Verification items for the finished model (mm, model axes). A direction names the side the tool comes from. Round coordinates to 2 decimals unless told otherwise and drop trailing zeros. Loops run counter-clockwise (first coordinate to the right, second up) from the corner with the lowest first, then second, coordinate; pieces in that order, holes last. Notation, with made-up numbers: (68.5, -1) -> (91.5, -1) arc R10 cw to (91.5, 6) -> close; hole circle Ø3 at (40, -5). An arc over 180 degrees is marked (long way). Write item = value, one per line.
Autodesk Inventor part; units mm, degrees
ref_plane "YZ Plane" through (0, 0, 0) normal (1, 0, 0) x (0, 1, 0)
ref_plane "XZ Plane" through (0, 0, 0) normal (0, 1, 0) x (-1, 0, 0)
ref_plane "XY Plane" through (0, 0, 0) normal (0, 0, 1) x (1, 0, 0)
sketch "Sketch1" plane through (0, 0, 0) normal (0, 1, 0) x (-1, 0, 0)
  line L0 (0, 21.535) -> (65.7, 21.535)
  line L1 (0, 21.535) -> (40.8722, -5.4921)
  line L2 (0, 21.535) -> (49, 21.535) construction
  line L3 (40.8722, -5.4921) -> (65.7, 21.535)
  line L4 (65.7, 21.535) -> (68.7, 21.535)
  line L5 (68.7, 21.535) -> (0, 21.535)
  line L6 (0, 21.535) -> (-3, 21.535)
  line L7 (40.8722, -5.4921) -> (43.3746, -7.1468)
  line L8 (65.7, 21.535) -> (38.8426, -7.7015)
  line L9 (137.4, 18.035) -> (137.4, 25.035)
  line L10 (137.4, 25.035) -> (0, 25.035)
  line L11 (0, 25.035) -> (0, 18.035)
  line L12 (0, 18.035) -> (137.4, 18.035)
  line L13 (137.4, 18.035) -> (0, 25.035) construction
  line L14 (137.4, 25.035) -> (0, 18.035) construction
  line L15 (93.1053, 46.1943) -> (87.9503, 50.9298)
  line L16 (87.9503, 50.9298) -> (38.2947, -3.1243)
  line L17 (38.2947, -3.1243) -> (43.4497, -7.8599)
  line L18 (43.4497, -7.8599) -> (93.1053, 46.1943)
  line L19 (93.1053, 46.1943) -> (38.2947, -3.1243) construction
  line L20 (87.9503, 50.9298) -> (43.4497, -7.8599) construction
  line L21 (79.8139, -35.4386) -> (83.6749, -29.5997)
  line L22 (83.6749, -29.5997) -> (1.9305, 24.4544)
  line L23 (1.9305, 24.4544) -> (-1.9305, 18.6155)
  line L24 (-1.9305, 18.6155) -> (79.8139, -35.4386)
  line L25 (79.8139, -35.4386) -> (1.9305, 24.4544) construction
  line L26 (83.6749, -29.5997) -> (-1.9305, 18.6155) construction
  line L27 (38.8426, -7.7015) -> (38.4743, -8.1025)
  line L28 (68.7, 21.535) -> (68.7, 25.035)
  line L29 (68.7, 21.535) -> (68.7, 18.035)
  line L30 (0, 25.035) -> (-3, 25.035)
  line L31 (-3, 25.035) -> (-3, 18.035)
  line L32 (-3, 18.035) -> (0, 18.035)
  line L33 (50.67, 0) -> (41.4309, -10.0576)
  circle A0 centre (65.7, 21.535) radius 1.65
  circle A1 centre (40.8722, -5.4921) radius 1.65
  circle A2 centre (0, 21.535) radius 1.65
  point P0 (0, 0)
  point P1 (40.3135, -0.9267)
  point P2 (11.6384, 18.035)
  point P3 (57.7322, 18.035)
  point P4 (-1.0525, 18.035)
  point P5 (73.6678, 25.035)
  dimension "d0" = 65.7
  dimension "d2" = 33.475
  dimension "d3" = 3
  dimension "d4" = 3
  dimension "d7" = 39.7
  dimension "d8" = 7
  dimension "d9" = 7
  dimension "d10" = 7
  dimension "d11" = 3.3
  dimension "d12" = 3.3
  dimension "d13" = 3.3
extrude "Extrusion1" add sketch "Sketch1" along normal blind 5 contours A2 L23 L22 L0 | L0 L22 L12 L1 A2 | L1 L12 L11 A2 | A2 L23 L24 L32 L31 L6 | L6 L31 L30 L11 A2 | L11 L10 L16 L0 L22 L23 A2 | L11 L32 L24 L23 A2 | L0 L16 L12 L22 | L12 L22 L16 L17 A1 L1 | L1 A1 L8 L27 L24 L32 L12 | L16 L10 L28 L4 A0 L0 | L0 A0 L3 L12 L16 | L12 L3 L22 L16 | L22 L3 A1 L17 L16 | A1 L17 L33 L24 L27 L8 | L10 L18 L29 L28 | L4 L29 L18 L12 L3 A0 | L12 L18 L22 L3 | L22 L18 L17 A1 L3
sketch "Sketch2" plane through (0, 5, 0) normal (0, 1, 0) x (1, 0, 0)
  line L0 (1.0525, -18.035) -> (-41.4309, 10.0576)
  line L1 (-41.4309, 10.0576) -> (11.6284, -25.035)
  line L2 (-41.4309, 10.0576) -> (22.1833, 10.0576) construction
  line L3 (-73.6678, -25.035) -> (3, -25.035)
  line L4 (11.6284, -25.035) -> (3, -25.035)
  line L5 (3, -25.035) -> (3, -18.035)
  line L6 (3, -18.035) -> (3, -25.035)
  point P0 (0, 0)
  point P1 (3, -19.3283)
  dimension "d16" = 33.48
extrude "Extrusion2" add sketch "Sketch2" against normal up to surface (5 mm away)
sketch "Sketch3" plane through (0, 5, 0) normal (0, 1, 0) x (1, 0, 0)
  line L0 (3, -18.035) -> (1.0525, -18.035)
  line L1 (11.6284, -25.035) -> (3, -19.3283)
  line L2 (1.0525, -18.035) -> (3, -19.3283)
  line L3 (3, -19.3283) -> (3, -18.035)
  line L4 (3, -18.035) -> (1.0525, -18.035)
  point P0 (0, 0)
extrude "Extrusion3" cut sketch "Sketch3" against normal blind 10
fillet "Fillet1" radius 3.5875 2 edges at (-73.6678, 2.5, 25.035) (-41.4309, 2.5, -10.0576)
fillet "Fillet2" radius 3.5875 1 edges at (11.6284, 2.5, 25.035)
properties part number "ghi"
(1) Sectioned sample at B-B, the plane x = -31. Record the cut outline in (y, z) (3 decimals), and give its area (3 significant figures).
Filled sheet:
outline = (0, -3.16) -> (5, -3.16) -> (5, 5.232) -> (0, 5.232) -> close; (0, 18.035) -> (5, 18.035) -> (5, 25.035) -> (0, 25.035) -> close
area = 77.0 mm2
(2) Draft check along X on faces 1 (the face through (-33, 5, 19)), 2 (the face through (2.01, 2.54, 18.67)), 3 (the face through (-64.39, 2.46, 22.54)). Enter one of: released by +X, released by -X, zero draft, split by the parting line, or undercut.
Filled sheet:
face_1 = zero draft
face_2 = released by +X
face_3 = undercut
(3) Material ranges on probe 1 along X at (y, z) = (2.75, 21.5); probe 2 along Z at (x, y) = (-45, 2.45) (3 decimals); probe 3 along X at (y, z) = (0.75, 5), recorded low to high. Write a range as from..to.
Filled sheet:
probe_1 = -69.09..-67.35, -64.05..-1.65, 1.65..3.69
probe_2 = -6.172..4.175, 18.035..25.035
probe_3 = -55.26..-45.76, -31.35..-18.66
(4) Set-up check for faces 4 (the face through (-33, 0, 19)), 5 (the face through (-34, 2, 18.035)): record each of +Z, -Z, +X, -X, +Y, -Y from which the full face is reachable in a straight line by a thin tool's end or side.
Filled sheet:
face_4 = +Z, -Z, +X, -X, -Y
face_5 = +Y, -Y
(5) Go/stop test with flat-tipped pins: pin 1 Ø1 at (y, z) = (1.5, -1) entering from -X; pin 2 Ø2 at (y, z) = (1, 8) entering from +X; pin 3 Ø2 at (x, z) = (0, 21.535) entering from -Y; pin 4 Ø1.5 at (x, y) = (-33, 2.5) entering from -Z. Record where each tip stops, or that it passes through.
Filled sheet:
pin_1 = -50.21
pin_2 = -12.61
pin_3 = through
pin_4 = -4.98
(6) Sectioned sample at C-C, the plane y = 1.45. Count the separate pieces of the cut face and the enclosed holes in it, and give its area (3 significant figures).
Filled sheet:
separate_pieces = 1
enclosed_holes = 4
area = 994 mm2
(7) Sectioned sample at D-D, the plane x = -5. Record the cut outline in (y, z) (3 decimals).
Filled sheet:
outline = (0, 14.033) -> (5, 14.033) -> (5, 25.035) -> (0, 25.035) -> close
(8) Sectioned sample at A-A, the plane z = 0. Record the cut outline in (x, y).
Filled sheet:
outline = (-50.67, 0) -> (-41.16, 0) -> (-41.16, 5) -> (-50.67, 5) -> close; (-38.91, 0) -> (-26.22, 0) -> (-26.22, 5) -> (-38.91, 5) -> close
